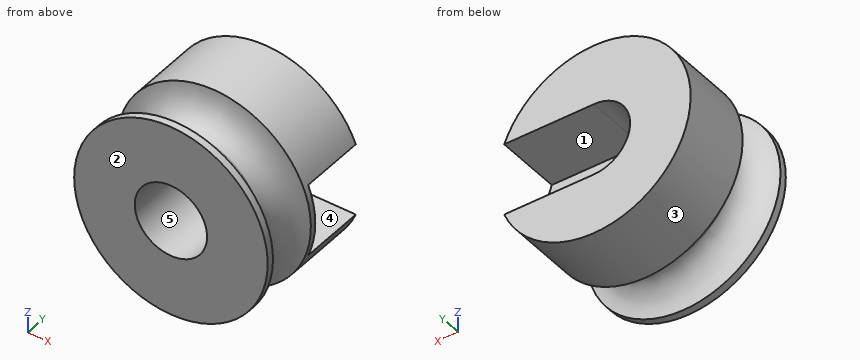
from build123d import *
from build123d.topology import SkipClean

# Parameters (mm, degrees)
SKETCH1_R               = 7.35
BOSS_EXTRUDE1_DEPTH     = 10
CUT_EXTRUDE1_DEPTH      = 5
CUT_EXTRUDE2_DEPTH      = 15.423765112
CUT_EXTRUDE2_DEPTH_BACK = 15.423765112
SKETCH3_R               = 2.75
SKETCH4_RX              = 2.5
SKETCH4_RY              = 2


with BuildPart() as part:
    # Sketch1 → Boss-Extrude1 (new body)
    with BuildSketch(Plane(origin=(0, 0, 0), x_dir=(1, 0, 0), z_dir=(0, 1, 0))):
        with Locations(Location((0, 0, 0), (0, 0, 270))):
            Circle(SKETCH1_R)
    extrude(amount=BOSS_EXTRUDE1_DEPTH)

    # Sketch2 → Cut-Extrude1 (cut)
    with BuildSketch(Plane(origin=(0, 10, 0), x_dir=(1, 0, 0), z_dir=(0, 1, 0))):
        with BuildLine():
            Line((0, 2.75), (9.425049625, 2.75))
            Line((9.425049625, 2.75), (9.711324497, -2.75))
            Line((9.711324497, -2.75), (0, -2.75))
            ThreePointArc((0, -2.75), (-2.75, 0), (0, 2.75))
        make_face()
    extrude(amount=-CUT_EXTRUDE1_DEPTH, mode=Mode.SUBTRACT)

    # Sketch3 → Cut-Extrude2 (cut, two sides: drawn at the far end of the back side and taken through both)
    with BuildSketch(Plane(origin=(0, 10, 0), x_dir=(1, 0, 0), z_dir=(0, 1, 0)).offset(-CUT_EXTRUDE2_DEPTH_BACK)):
        with Locations(Location((0, 0, 0), (0, 0, 270))):
            Circle(SKETCH3_R)
    extrude(amount=CUT_EXTRUDE2_DEPTH + CUT_EXTRUDE2_DEPTH_BACK, mode=Mode.SUBTRACT)

    # Sketch4 → Cut-Revolve1 (revolve, cut)
    with SkipClean():  # the faces are left unmerged after this step: merging them gives an invalid solid
        with BuildSketch(Plane.XY, mode=Mode.PRIVATE) as cut_revolve1_sk:
            with Locations((-7.59796792, 2.550632184)):
                Ellipse(SKETCH4_RX, SKETCH4_RY)
        revolve(cut_revolve1_sk.sketch.rotate(Axis((0, 10, 0), (0, 1, 0)), 270), axis=Axis((0, 10, 0), (0, 1, 0)), mode=Mode.SUBTRACT)


solid = part.part
Read the model definition and answer for the solid it produces. Units are mm, in the model's axes. Face numbers are marked on the shaded views. A direction names the side the tool comes from. Give positions to 0.01 mm unless a question says otherwise; leave off trailing zeros. Loops run counter-clockwise (first coordinate to the right, second up) from the corner with the lowest first, then second, coordinate; pieces in that order, holes last. Notation, with made-up numbers: (0, 36) -> (41, 36) arc R25 cw to (41, 73) -> close; hole circle Ø5 at (44, 62). An arc over 180 degrees is marked (long way). Use a Markdown table: item, result.
Q1. Section A-A, the plane y = 5.25 is taken. Determine the outline of the cut face in (x, z), then the cut area to 3 significant figures.
Solved:
| item | result |
|---|---|
| outline | (0, -2.75) arc R2.75 cw to (0, 2.75) -> (6.82, 2.75) arc R7.35 ccw (long way) to (6.82, -2.75) -> close |
| area | 118 mm^2 |
Q2. Determine the mould class of the marked faces 1, 2 and 3 for opening direction Z: pulls with the +Z half, pulls with the -Z half, needs draft (parallel to the pull), parting line crosses it, or undercut.
Solved:
| item | result |
|---|---|
| face 1 | undercut |
| face 2 | needs draft |
| face 3 | parting line crosses it |
Q3. A tool of negligible diameter and unlimited length cuts with its end or side. For the marked faces 4 and 5, from which of +Z, -Z, +X, -X, +Y, -Y can it reach the whole face along a straight path? Write none if from no direction.
Solved:
| item | result |
|---|---|
| face 4 | +X, +Y |
| face 5 | +Y, -Y |
Q4. Find the intervals of material crossed by line 1 along Z through (x, y) = (0, 6); line 2 along Y through (x, z) = (3.75, -2); line 3 along Y through (x, z) = (4.5, 4.25), in increasing order.
Solved:
| item | result |
|---|---|
| line 1 | z = -7.35 to -2.75, 2.75 to 7.35 |
| line 2 | y = 0 to 5 |
| line 3 | y = 0 to 0.9, 4.2 to 10 |
Q5. Each of these flat-tipped pins is pushed along its axis until it touches: pin 1 (2.5 mm diameter, centred on x = 4, y = 8.5, fed in from -Z); pin 2 (4 mm diameter, centred on x = 4.5, y = 6, fed in from +Z); pin 3 (4 mm diameter, centred on x = 4, y = 8, fed in from +Z). Where does it stop, or does it pass through?
Solved:
| item | result |
|---|---|
| pin 1 | stops at z = -6.82 |
| pin 2 | stops at z = 6.91 |
| pin 3 | stops at z = 7.07 |
